Work out the finished part from the listing and answer in its coordinate system (mm). A direction names the side the tool comes from. Round coordinates to 2 decimals unless told otherwise and drop trailing zeros. Order: outer loops, then holes, each group sorted by start corner. A loop starts at its lowest first (then second) coordinate and runs counter-clockwise, first axis right, second up. Notation, with made-up numbers: (12.25, -9.75) -> (58.25, -9.75) arc R28 cw to (58.25, 24.25) -> close; hole circle Ø10 at (-35, -21). An arc over 180 degrees is marked (long way). Use a Markdown table: item, result. Add a question column.
Item 1: A flat-ended cylindrical pin translates along its axis: P1, Ø1.5, axis at x = -4, y = -3.5, coming from the +Z side. Find the tip coordinate at first contact, or state that the pin passes through.
Item 2: A cutting plane is placed at D-D, the plane x = 2.5. Determine the outline of the cut face in (y, z), plus the area to 3 significant figures.
Item 3: For a pull along X with two mould halves and no side action, classify faces 1 (the flat face through (10, 0, 0)), 2 (the cylindrical face through (8.14, -4.05, -2.58)), 3 (the cylindrical face through (9.16, -4.88, 1.08)) as +X half, -X half, draft (parallel to the pull), parting line (faces both ways), or undercut.
Item 4: Find the intervals of material crossed by L1, parallel to X at y = 0, z = 4.2; L2, parallel to X at y = -3.5, z = 1; L3, parallel to Z at x = 1, y = -0.5, in increasing order. Write a range as [from, to].
Item 5: A cutting plane is placed at C-C, the plane x = 0. Determine the outline of the cut face in (y, z).
Item 6: A cutting plane is placed at B-B, the plane z = 0. Determine the outline of the cut face in (x, y), plus the area to 3 significant figures.
Item 7: A tool of negligible diameter and unlimited length cuts with its end or side. For faces 4 (the cylindrical face through (1.65, -0.07, -0.07)), 5 (the cylindrical face through (-8.14, -4.05, -2.58)), from which of +Z, -Z, +X, -X, +Y, -Y can it reach the whole face along a straight path? Write none if from no direction.
from build123d import *

# Parameters (mm, degrees)
SKETCH1_R           = 5
BOSS_EXTRUDE1_DEPTH = 10
SKETCH2_W           = 1.1
SKETCH2_H           = 0.2
CHAMFER1_SIZE       = 0.4
M4_TAPPED_HOLE4_D   = 3.3
SKETCH6_R           = 1
CUT_EXTRUDE1_DEPTH  = 16.0000001


with BuildPart() as part:
    # Sketch1 → Boss-Extrude1 (new, symmetric)
    with BuildSketch(Plane(origin=(0, 0, 0), x_dir=(0, 0, -1), z_dir=(1, 0, 0))):
        Circle(SKETCH1_R)
    extrude(amount=BOSS_EXTRUDE1_DEPTH, both=True)

    # Sketch2 → Cut-Revolve1 (revolve, cut)
    with BuildSketch(Plane(origin=(0, 0, 0), x_dir=(1, 0, 0), z_dir=(0, 1, 0))):
        with Locations((-8.15, 4.9)):
            Rectangle(SKETCH2_W, SKETCH2_H)
    cut_revolve1 = revolve(axis=Axis((0, 0, 0), (-1, 0, 0)), mode=Mode.SUBTRACT)

    # Mirror1: Cut-Revolve1 across plane
    add(cut_revolve1.mirror(Plane(origin=(0, 0, 0), x_dir=(0, 0, 1), z_dir=(1, 0, 0))), mode=Mode.SUBTRACT)

    # Chamfer1
    chamfer1_edges = [part.edges().sort_by_distance(p)[0] for p in [
        (-10, 0, 5),
        (10, 0, 5),
    ]]
    chamfer(chamfer1_edges, length=CHAMFER1_SIZE)

    # M4 Tapped Hole4 (through all)
    with Locations(Plane(origin=(0, 5, 0), x_dir=(1, 0, 0), z_dir=(0, 1, 0))):
        with Locations((0, 0)):
            Hole(M4_TAPPED_HOLE4_D / 2)

    # Sketch6 → Cut-Extrude1 (cut, through all)
    with BuildSketch(Plane(origin=(0, 0, -5), x_dir=(-1, 0, 0), z_dir=(0, 0, -1))):
        Circle(SKETCH6_R)
    extrude(amount=-CUT_EXTRUDE1_DEPTH, mode=Mode.SUBTRACT)


solid = part.part
Reported:
| question | item | result |
|---|---|---|
| 1 | P1 | z = 4.18 |
| 2 | outline | circle Ø10 at (0, 0) |
| 2 | area | 78.5 mm² |
| 3 | face 1 | +X half |
| 3 | face 2 | undercut |
| 3 | face 3 | draft |
| 4 | L1 | [-10, -1], [1, 10] |
| 4 | L2 | [-10, -1.31], [1.31, 10] |
| 4 | L3 | [-4.97, -1.31], [1.31, 4.97] |
| 5 | outline | (-4.72, -1.65) arc R5 ccw to (-1, -4.9) -> (-1, -1.65) -> close; (-4.72, 1.65) -> (-1, 1.65) -> (-1, 4.9) arc R5 ccw to start; (1, -4.9) arc R5 ccw to (4.72, -1.65) -> (1, -1.65) -> close; (1, 1.65) -> (4.72, 1.65) arc R5 ccw to (1, 4.9) -> close |
| 6 | outline | (-10, -4.6) -> (-9.6, -5) -> (-8.7, -5) -> (-8.7, -4.8) -> (-7.6, -4.8) -> (-7.6, -5) -> (-1.65, -5) -> (-1.65, 5) -> (-7.6, 5) -> (-7.6, 4.8) -> (-8.7, 4.8) -> (-8.7, 5) -> (-9.6, 5) -> (-10, 4.6) -> close; (1.65, -5) -> (7.6, -5) -> (7.6, -4.8) -> (8.7, -4.8) -> (8.7, -5) -> (9.6, -5) -> (10, -4.6) -> (10, 4.6) -> (9.6, 5) -> (8.7, 5) -> (8.7, 4.8) -> (7.6, 4.8) -> (7.6, 5) -> (1.65, 5) -> close |
| 6 | area | 166 mm² |
| 7 | face 4 | +Y, -Y |
| 7 | face 5 | none |
